Read the model definition and answer for the solid it produces. Units are mm, in the model's axes. Face numbers are marked on the shaded views. Coordinates: 2 decimals unless noted, no trailing zeros. Write each loop counter-clockwise with the first axis right and the second up, starting at its lowest first coordinate (ties: lowest second). Pieces come first, ordered by that corner, then holes. Notation, with made-up numbers: (68.5, -40) -> (84.5, -40) arc R28 ccw to (84.5, -22) -> close; hole circle Ø4 at (59.25, 58.25). An arc over 180 degrees is marked (long way). One line per item, written item: value. Start each with the question number.
1. Consider line 1 along Y through (x, z) = (0, -1.7); line 2 along Y through (x, z) = (-0.5, -2.8); line 3 along Y through (x, z) = (-3.5, -1.8). Determine where each line is inside the solid, lowest interval first.
2. Given P1, Ø1.9, axis at x = 0, y = 0, coming from the -Z side, flat-ended and moving along its own axis, determine where the tip first touches the part or whether it passes through.
3. Find section A-A, the plane x = 0. Write down the section's boundary in (y, z), and give its area (3 significant figures).
4. For a pull along Y with two mould halves and no side action, classify the marked faces 1, 2 and 3 as pulls with the +Y half, pulls with the -Y half, needs draft (parallel to the pull), parting line crosses it, or undercut.
5. Find section C-C, the plane x = 3. Write down the section's boundary in (y, z), and give its area (3 significant figures).
6. Find section D-D, the plane x = -2.75. Write down the section's boundary in (y, z), and give its area (3 significant figures).
7. Find section B-B, the plane z = -0.4. Write down the section's boundary in (x, y), and give its area (3 significant figures).
```python
from build123d import *

# Parameters (mm, degrees)
BOSS_EXTRUDE1_DEPTH = 3
SKETCH3_R           = 1.6
CUT_EXTRUDE1_DEPTH  = 4


with BuildPart() as part:
    # Sketch1 → Boss-Extrude1 (new body)
    with BuildSketch(Plane.XY):
        with BuildLine():
            Line((-4, 0), (-4, 40))
            ThreePointArc((-4, 40), (0, 44), (4, 40))
            Line((4, 40), (4, 0))
            ThreePointArc((4, 0), (0, -4), (-4, 0))
        make_face()
    extrude(amount=-BOSS_EXTRUDE1_DEPTH)

    # Sketch3 → Cut-Extrude1 (cut, through all)
    with BuildSketch(Plane.XY):
        Circle(SKETCH3_R)
        with Locations((0, 40)):
            Circle(SKETCH3_R)
    extrude(amount=-CUT_EXTRUDE1_DEPTH, mode=Mode.SUBTRACT)


solid = part.part
```
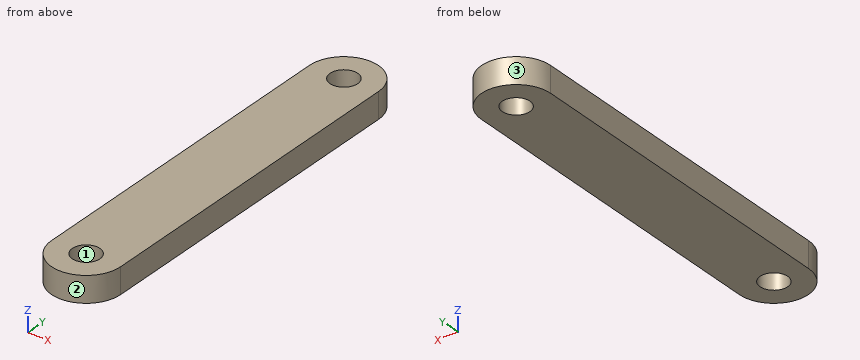
Answer block:
1. line 1: y = -4 to -1.6, 1.6 to 38.4, 41.6 to 44
1. line 2: y = -3.97 to -1.52, 1.52 to 38.48, 41.52 to 43.97
1. line 3: y = -1.94 to 41.94
2. P1: passes through
3. outline: (-4, -3) -> (-1.6, -3) -> (-1.6, 0) -> (-4, 0) -> close; (1.6, -3) -> (38.4, -3) -> (38.4, 0) -> (1.6, 0) -> close; (41.6, -3) -> (44, -3) -> (44, 0) -> (41.6, 0) -> close
3. area: 125 mm2
4. face 1: undercut
4. face 2: pulls with the -Y half
4. face 3: pulls with the +Y half
5. outline: (-2.65, -3) -> (42.65, -3) -> (42.65, 0) -> (-2.65, 0) -> close
5. area: 136 mm2
6. outline: (-2.9, -3) -> (42.9, -3) -> (42.9, 0) -> (-2.9, 0) -> close
6. area: 137 mm2
7. outline: (-4, 0) arc R4 ccw to (4, 0) -> (4, 40) arc R4 ccw to (-4, 40) -> close; hole circle Ø3.2 at (0, 0); hole circle Ø3.2 at (0, 40)
7. area: 354 mm2
